Geometry: final body of the model. Coordinates: model frame, mm. Face numbers are marked on the shaded views. Give positions to 0.01 mm unless a question says otherwise; leave off trailing zeros. Order: outer loops, then holes, each group sorted by start corner. A loop starts at its lowest first (then second) coordinate and runs counter-clockwise, first axis right, second up. Notation, with made-up numbers: (44.5, 70) - (48.5, 70) arc R16 ccw to (48.5, 86) - close; hole circle Ø3 at (16, -35.75). An arc over 180 degrees is marked (long way). Put each result on its own line as item: value. Start each with the question number.
1. Mould query, pull axis Y, two halves, no side actions, for the marked faces 1, 2 and 3. Classes: pulls with the +Y half, pulls with the -Y half, needs draft (parallel to the pull), parting line crosses it, or undercut.
2. Section B-B on z = -3.25. Return the cut outline in (x, y).
3. Section A-A on z = -5.25. Return the cut outline in (x, y), plus the area to 3 significant figures.
4. First-contact query: P1, Ø3, axis at x = 1, z = -4, coming from the +Y side; P2, Ø1, axis at x = -2.5, z = -4, coming from the -Y side; P3, Ø1.2, axis at x = 0, y = 0, coming from the +Z side. Flat tips, straight axial feed; report the tip coordinate or a pass-through.
5. Ray query, line 1 along Y through (x, z) = (0, -6.7); line 2 along Y through (x, z) = (-0.5, -5); line 3 along X through (y, z) = (-1, -0.5). Return the intervals inside material, ascending. Write a range as from..to.
Autodesk Inventor part; units mm, degrees
ref_plane "Work Plane1" through (0, 0, -7.5) normal (0, 0, 1) x (1, 0, 0)
ref_plane "YZ Plane" through (0, 0, 0) normal (1, 0, 0) x (0, 1, 0)
ref_plane "XZ Plane" through (0, 0, 0) normal (0, 1, 0) x (-1, 0, 0)
sketch "Sketch1" plane through (0, 0, 0) normal (0, 0, 1) x (1, 0, 0)
  circle A0 centre (0, 0) radius 5
  dimension "d0" = 10
ref_plane "Work Plane1" through (0, 0, -7.5) normal (0, 0, 1) x (1, 0, 0)
sketch "Sketch2" plane through (0, 0, -7.5) normal (0, 0, 1) x (1, 0, 0)
  circle A0 centre (0, 0) radius 2.5
  dimension "d2" = 5
loft "Loft1" add profiles "Sketch1", "Sketch2"
sketch "Sketch3" plane through (0, 0, 0) normal (0, 1, 0) x (-1, 0, 0)
  arc A0 (0, 2.5) -> (0, -4.5) centre (0, -1) ccw
  line L0 (0, 5.5184) -> (0, -9.2276)
  line L1 (2.5, -7.5) -> (-2.5, -7.5)
  point P0 (0, 0)
  dimension "d7" = 7
  dimension "d9" = 1
revolve "Revolution1" cut sketch "Sketch3" angle 360 about axis through (0, 0, 5.5184) along (0, 0, -1)
sketch "Sketch4" plane through (0, 0, -7.5) normal (0, 0, -1) x (-1, 0, 0)
  circle A0 centre (0, 0) radius 1
  dimension "d10" = 2
extrude "Extrusion1" cut sketch "Sketch4" against normal blind 3
properties part number "Socket"
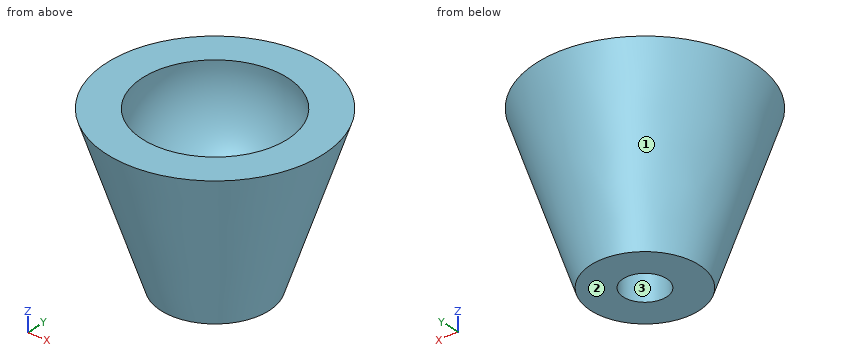
Resolved:
1. face 1: parting line crosses it
1. face 2: needs draft
1. face 3: undercut
2. outline: circle Ø7.83 at (0, 0); hole circle Ø5.36 at (0, 0)
3. outline: circle Ø6.5 at (0, 0); hole circle Ø2 at (0, 0)
3. area: 30.0 mm^2
4. P1: y = 4.11
4. P2: y = -3.13
4. P3: z = -4.45
5. line 1: -2.77..-1, 1..2.77
5. line 2: -3.3..-0.87, 0.87..3.3
5. line 3: -4.73..-3.32, 3.32..4.73
